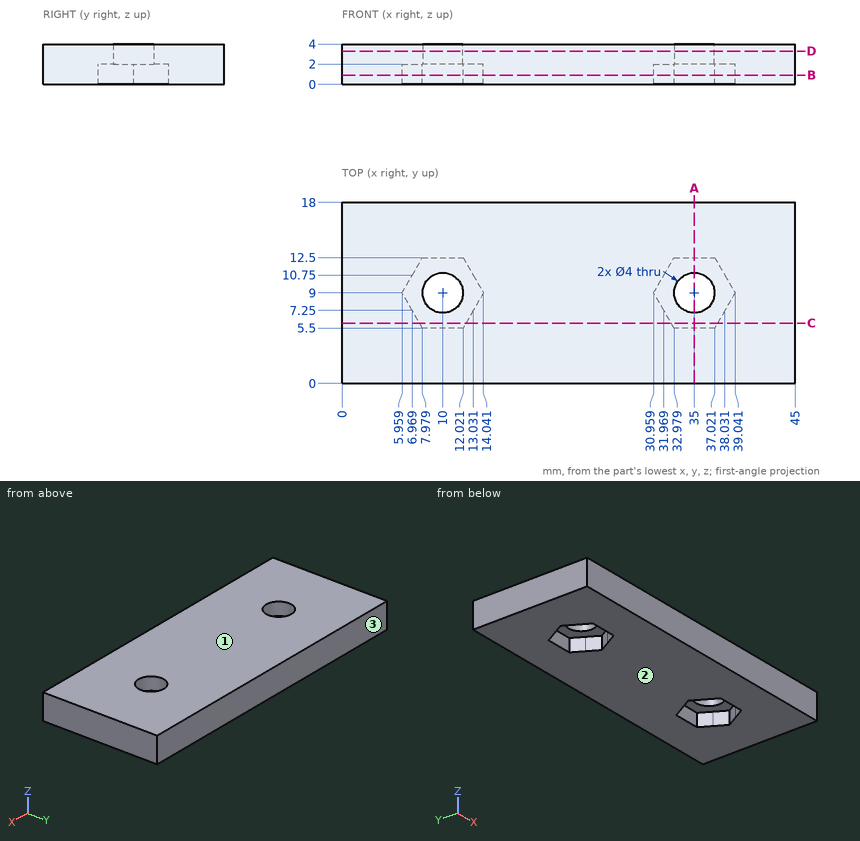
Answer from the drawing. Dimensions are ordinates in mm from the lowest x, y and z of the part. Give positions to 0.01 mm unless a question says otherwise; leave off trailing zeros. Write each loop counter-clockwise with the first axis right and the second up, starting at its lowest first coordinate (ties: lowest second). Pieces come first, ordered by that corner, then holes. Notation, with made-up numbers: (-4.75, -39.75) -> (21.25, -39.75) arc R11 cw to (21.25, -25.75) -> close; hole circle Ø11 at (-28, -1.5). An arc over 180 degrees is marked (long way). One line per question, with ' | ' between items. Start each with the question number.
1. Find the intervals of material crossed by probe 1 along X at (y, z) = (9, 3); probe 2 along Y at (x, z) = (10.5, 0.4); probe 3 along Y at (x, z) = (10, 3.5), in increasing order.
2. Section C-C (y = 6) is taken. Determine the outline of the cut face in (x, z).
3. For a pull along Z with two mould halves and no side action, classify the marked faces 1, 2 and 3 as pulls with the +Z half, pulls with the -Z half, needs draft (parallel to the pull), parting line crosses it, or undercut.
4. Section A-A (x = 35) is taken. Determine the outline of the cut face in (y, z), plus the area to 3 significant figures.
5. Given pin 1 Ø2 at (x, y) = (9, 10) entering from -Z; pin 2 Ø5 at (x, y) = (23, 4) entering from -Z, each flat-ended and moving along its own axis, determine where each tip first touches the part or whether it passes through.
6. Section B-B (z = 0.9) is taken. Determine the outline of the cut face in (x, y), plus the area to 3 significant figures.
7. Section D-D (z = 3.3) is taken. Determine the outline of the cut face in (x, y), plus the area to 3 significant figures.
Response values:
1) probe 1: 0 to 8, 12 to 33, 37 to 45 | probe 2: 0 to 5.5, 12.5 to 18 | probe 3: 0 to 7, 11 to 18
2) outline: (0, 0) -> (7.69, 0) -> (7.69, 2) -> (12.31, 2) -> (12.31, 0) -> (32.69, 0) -> (32.69, 2) -> (37.31, 2) -> (37.31, 0) -> (45, 0) -> (45, 4) -> (0, 4) -> close
3) face 1: pulls with the +Z half | face 2: pulls with the -Z half | face 3: needs draft
4) outline: (0, 0) -> (5.5, 0) -> (5.5, 2) -> (7, 2) -> (7, 4) -> (0, 4) -> close; (11, 2) -> (12.5, 2) -> (12.5, 0) -> (18, 0) -> (18, 4) -> (11, 4) -> close | area: 50.0 mm2
5) pin 1: z = 2 | pin 2: z = 0
6) outline: (0, 0) -> (45, 0) -> (45, 18) -> (0, 18) -> close; hole (5.96, 9) -> (7.98, 5.5) -> (12.02, 5.5) -> (14.04, 9) -> (12.02, 12.5) -> (7.98, 12.5) -> close; hole (30.96, 9) -> (32.98, 5.5) -> (37.02, 5.5) -> (39.04, 9) -> (37.02, 12.5) -> (32.98, 12.5) -> close | area: 725 mm2
7) outline: (0, 0) -> (45, 0) -> (45, 18) -> (0, 18) -> close; hole circle Ø4 at (10, 9); hole circle Ø4 at (35, 9) | area: 785 mm2
